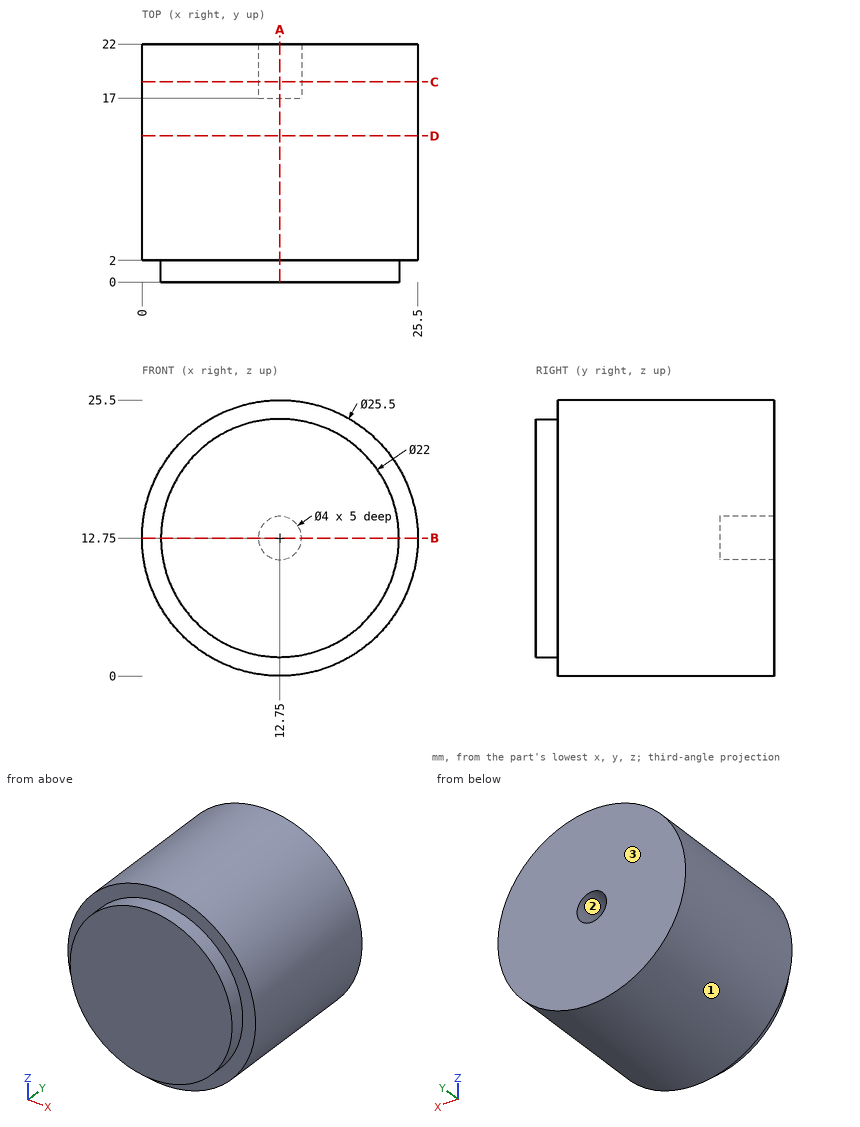
Can you work these out from the drawing? Everything is in mm from the part's minimum corner. Coordinates: 2 decimals unless noted, no trailing zeros. Loops run counter-clockwise (first coordinate to the right, second up) from the corner with the lowest first, then second, coordinate; pieces in that order, holes last. Notation, with made-up numbers: (44, -3) - (92, -3) arc R27 ccw to (92, 26) - close; hole circle Ø5 at (83.25, -19.75). An arc over 180 degrees is marked (long way). Use a Markdown table: item, result.
Item 1: I want a section at D-D on y = 13.5. Please give me the cut outline in (x, z), and give its area (3 significant figures).
Numbers:
| item | result |
|---|---|
| outline | circle Ø25.5 at (12.75, 12.75) |
| area | 511 mm2 |
Item 2: We'd pull the mould along Z, two halves only. Please class the marked faces 1, 2 and 3: released by +Z, released by -Z, zero draft, split by the parting line, or undercut.
Numbers:
| item | result |
|---|---|
| face 1 | split by the parting line |
| face 2 | undercut |
| face 3 | zero draft |
Item 3: Will these pins go through, and if not, where does the flat tip stop? pin 1 (1 mm diameter, centred on x = 15.5, y = 6.5, fed in from +Z); pin 2 (1 mm diameter, centred on x = 22.5, z = 22, fed in from -Y); pin 3 (5 mm diameter, centred on x = 5.5, y = 8, fed in from +Z); pin 4 (12 mm diameter, centred on y = 17, z = 19, fed in from +X).
Numbers:
| item | result |
|---|---|
| pin 1 | stops at z = 25.3 |
| pin 2 | passes through |
| pin 3 | stops at z = 24.58 |
| pin 4 | stops at x = 25.5 |
Item 4: I want a section at B-B on z = 12.75. Please give me the cut outline in (x, y), and give its area (3 significant figures).
Numbers:
| item | result |
|---|---|
| outline | (0, 2) - (1.75, 2) - (1.75, 0) - (23.75, 0) - (23.75, 2) - (25.5, 2) - (25.5, 22) - (14.75, 22) - (14.75, 17) - (10.75, 17) - (10.75, 22) - (0, 22) - close |
| area | 534 mm2 |
Item 5: I want a section at A-A on x = 12.75. Please give me the cut outline in (y, z).
Numbers:
| item | result |
|---|---|
| outline | (0, 1.75) - (2, 1.75) - (2, 0) - (22, 0) - (22, 10.75) - (17, 10.75) - (17, 14.75) - (22, 14.75) - (22, 25.5) - (2, 25.5) - (2, 23.75) - (0, 23.75) - close |
Item 6: I want a section at C-C on y = 18.5. Please give me the cut outline in (x, z), and give its area (3 significant figures).
Numbers:
| item | result |
|---|---|
| outline | circle Ø25.5 at (12.75, 12.75); hole circle Ø4 at (12.75, 12.75) |
| area | 498 mm2 |
Item 7: If I drill on probe 1 along Z at (x, y) = (12.75, 20.7); probe 2 along Y at (x, z) = (1.75, 15); probe 3 along X at (y, z) = (9.5, 13.5), over which ranges is the centre line in solid material (lowest first)? Write a range as from..to.
Numbers:
| item | result |
|---|---|
| probe 1 | z = 0..10.75, 14.75..25.5 |
| probe 2 | y = 2..22 |
| probe 3 | x = 0.02..25.48 |
